Design review of the part built by this model. Coordinates are the model's own, in mm. A direction names the side the tool comes from. Coordinates: 2 decimals unless noted, no trailing zeros. Loops run counter-clockwise (first coordinate to the right, second up) from the corner with the lowest first, then second, coordinate; pieces in that order, holes last. Notation, with made-up numbers: M 39,24.5 L 63,24.5 A26 ccw 63,49.5 Z; hole C 44,-21.5 d4. An arc over 180 degrees is marked long. Answer as CSV lines item,"result". Start each with the question number.
Autodesk Inventor part; units mm, degrees
ref_plane "YZ Plane" through (0, 0, 0) normal (1, 0, 0) x (0, 1, 0)
ref_plane "XZ Plane" through (0, 0, 0) normal (0, 1, 0) x (-1, 0, 0)
ref_plane "XY Plane" through (0, 0, 0) normal (0, 0, 1) x (1, 0, 0)
sketch "草圖1" plane through (0, 0, 0) normal (0, 0, 1) x (1, 0, 0)
  line L0 (0, 0) -> (-30, 0)
  line L1 (-30, 0) -> (-30, 50)
  line L2 (-30, 50) -> (0, 50)
  line L3 (0, 50) -> (0, 0)
  line L4 (-30, 0) -> (-70, 0)
  line L5 (-70, 0) -> (-70, 30)
  line L6 (-70, 30) -> (-30, 30)
  line L7 (-30, 30) -> (-30, 0)
  line L8 (-70, 0) -> (-150, 0)
  line L9 (-150, 0) -> (-150, 10)
  line L10 (-150, 10) -> (-70, 10)
  line L11 (-70, 10) -> (-70, 0)
  dimension "d0" = 30
  dimension "d1" = 40
  dimension "d2" = 80
  dimension "d3" = 10
  dimension "d4" = 30
  dimension "d5" = 50
revolve "迴轉1" add sketch "草圖1" angle 360 about axis through (-70, 0, 0) along (-1, 0, 0)
mirror "鏡射1" about plane through (0, 0, 0) normal (1, 0, 0) of "迴轉1"
properties part number "P1"
Item 1: Add section C-C (x = 89). Give the boundary of the cut face in (y, z).
Item 2: For faces 1 (the face through (-0.42, 47.69, -15.02)), 2 (the face through (-109.44, -2.17, -9.76)), 3 (the face through (30, -22, 22)), list the 3-axis set-ups (+Z, -Z, +X, -X, +Y, -Y) from which the entire face can be reached by the end or side of a thin tool; tool diameter is ignored.
Item 3: Add section D-D (z = 25). Give the boundary of the cut face in (x, y).
Item 4: For pin 1 (1 mm diameter, centred on x = 29, z = -37, fed in from +Y); pin 2 (12 mm diameter, centred on y = 31.5, z = -29.5, fed in from -X); pin 3 (4 mm diameter, centred on y = 22, z = -8.5, fed in from -X); pin 4 (12 mm diameter, centred on x = 102, y = -18.5, fed in from -Z), all flat-tipped, find the tip position at first contact; note any pin that passes through.
Item 5: For line 1 along X through (y, z) = (-7.5, 43); line 2 along X through (y, z) = (18, 14.5); line 3 along Y through (x, z) = (19.5, -8), list the stretches that pass through material, from the lowest coordinate up. Write a range as from..to.
Item 6: Add section A-A (z = 0). Give the boundary of the cut face in (x, y).
Response:
1,outline,"C 0,0 d20"
2,face 1,"+X, -X"
2,face 2,"-X"
2,face 3,"+X"
3,outline,"M -70,-16.58 L -30,-16.58 L -30,-43.3 L 30,-43.3 L 30,-16.58 L 70,-16.58 L 70,16.58 L 30,16.58 L 30,43.3 L -30,43.3 L -30,16.58 L -70,16.58 Z"
4,pin 1,"y = 34.17"
4,pin 2,"x = -30"
4,pin 3,"x = -70"
4,pin 4,"through"
5,line 1,"-30..30"
5,line 2,"-70..70"
5,line 3,"-49.36..49.36"
6,outline,"M -150,-10 L -70,-10 L -70,-30 L -30,-30 L -30,-50 L 30,-50 L 30,-30 L 70,-30 L 70,-10 L 150,-10 L 150,10 L 70,10 L 70,30 L 30,30 L 30,50 L -30,50 L -30,30 L -70,30 L -70,10 L -150,10 Z"
